from build123d import *

# Parameters (mm, degrees)
F1_DEPTH = 19.05
F2_R     = 8.5
F3_DEPTH = 3.175
F4_R     = 4.5
F5_DEPTH = 15.875
F6_R     = 8.5
F7_DEPTH = 3.175
F8_SIZE  = 0.508


with BuildPart() as f1:
    # F0 (on Front) → F1 (new body)
    with BuildSketch(Plane.XZ):
        Polygon((-30, -16), (0, -16), (30, -16), (30, 7.6738381025), (17.8103312015, 7.6746507471), (17.810886279, 16.0008126076), (0, 16.002), (-17.810886279, 16.0008126076), (-17.8103312015, 7.6746507471), (-30, 7.6738381025), align=None)
    extrude(amount=F1_DEPTH)

    # F2 (on face) → F3 (cut)
    with BuildSketch(Plane.XZ.offset(19.05)):
        Circle(F2_R)
    extrude(amount=-F3_DEPTH, mode=Mode.SUBTRACT)

    # F4 (on face) → F5 (cut, through all)
    with BuildSketch(Plane.XZ.offset(15.875)):
        Circle(F4_R)
    extrude(amount=-F5_DEPTH, mode=Mode.SUBTRACT)

    # F6 (on Front) → F7 (cut)
    with BuildSketch(Plane.XZ):
        Circle(F6_R)
    extrude(amount=F7_DEPTH, mode=Mode.SUBTRACT)

    # F8
    f8_edges = [f1.edges().sort_by_distance(p)[0] for p in [
        (-30, -9.525, 7.673838),
        (-17.810886, -9.525, 16.000813),
        (-30, -19.05, -4.163081),
        (-8.905443, -19.05, 16.001406),
        (8.905443, -19.05, 16.001406),
        (23.905166, -19.05, 7.674244),
        (30, -19.05, -4.163081),
        (0, -19.05, -16),
        (-8.905443, 0, 16.001406),
        (8.905443, 0, 16.001406),
        (17.810886, -9.525, 16.000813),
        (-30, 0, -4.163081),
        (30, 0, -4.163081),
        (0, 0, -16),
        (30, -9.525, -16),
        (-30, -9.525, -16),
        (-8.5, 0, 0),
        (-23.905166, -19.05, 7.674244),
        (-17.810609, -19.05, 11.837732),
        (17.810609, -19.05, 11.837732),
        (-8.5, -19.05, 0),
    ]]
    chamfer(f8_edges, length=F8_SIZE)


solid = f1.part
The model under review builds one solid part; all positions refer to its coordinate system, in mm. A direction names the side the tool comes from. Coordinates: 2 decimals unless noted, no trailing zeros. Loops run counter-clockwise (first coordinate to the right, second up) from the corner with the lowest first, then second, coordinate; pieces in that order, holes last. Notation, with made-up numbers: M -13.5,-21.75 L 10.5,-21.75 A24 ccw 10.5,7.25 Z; hole C -35,46 d11. An arc over 180 degrees is marked long. Put each result on its own line as item: value. Start each with the question number.
Q1. Add section B-B (z = 0). Write out the cut boundary in (x, y) (3 decimals).
Q2. Wall thickness on line 1 (Z direction, x = 0, y = -2.3); line 2 (Z direction, x = 0, y = -6); line 3 (Z direction, x = 18.5, y = -6): over which ranges is each line inside the solid? List them lowest first.
Q3. Clearance check with flat-ended pins moving along their axes: pin 1 (5 mm diameter, centred on x = 4, z = 2, fed in from -Y) (3 decimals); pin 2 (13.5 mm diameter, centred on x = -3, z = 1.5, fed in from +Y); pin 3 (8 mm diameter, centred on y = -8.5, z = 12.5, fed in from -X); pin 4 (8 mm diameter, centred on x = 0, z = 0, fed in from +Y). State where each tip first meets the part, or that it passes through.
Q4. Add section A-A (y = -6). Write out the cut boundary in (x, z), and give its area (3 significant figures).
Q5. The part is to be moulded in two halves that separate along Z. For faces 1 (the flat face through (0, -9, -16)), 2 (the flat face through (4, -15.875, -4)), 3 (the flat face through (4, -3.175, -4)), 4 (the flat face through (-30, -9, -4)), say which applies: +Z half, -Z half, draft (parallel to the pull), parting line (faces both ways), or undercut.
Q6. For faces 5 (the cylindrical face through (-0.59, -9.61, 4.46)), 6 (the cylindrical face through (4.57, -17.227, 7.167)), 7 (the cylindrical face through (4.57, -1.823, 7.167)), list the 3-axis set-ups (+Z, -Z, +X, -X, +Y, -Y) from which the entire face can be reached by the end or side of a thin tool; tool diameter is ignored.
Q7. Add section C-C (x = 26.5). Write out the cut boundary in (y, z).
Answers:
1. outline: M -30,-18.542 L -29.492,-19.05 L -9.008,-19.05 L -8.5,-18.542 L -8.5,-15.875 L -4.5,-15.875 L -4.5,-3.175 L -8.5,-3.175 L -8.5,-0.508 L -9.008,0 L -29.492,0 L -30,-0.508 Z; M 4.5,-15.875 L 8.5,-15.875 L 8.5,-18.542 L 9.008,-19.05 L 29.492,-19.05 L 30,-18.542 L 30,-0.508 L 29.492,0 L 9.008,0 L 8.5,-0.508 L 8.5,-3.175 L 4.5,-3.175 Z
2. line 1: z = -16 to -8.5, 8.5 to 16
2. line 2: z = -16 to -4.5, 4.5 to 16
2. line 3: z = -16 to 7.67
3. pin 1: stops at y = -15.875
3. pin 2: stops at y = 0
3. pin 3: stops at x = -17.81
3. pin 4: passes through
4. outline: M -30,-15.49 L -29.49,-16 L 29.49,-16 L 30,-15.49 L 30,7.67 L 17.81,7.67 L 17.81,15.49 L 17.3,16 L 0,16 L -17.3,16 L -17.81,15.49 L -17.81,7.67 L -29.49,7.67 L -30,7.17 Z; hole C 0,0 d9
4. area: 1,650 mm^2
5. face 1: -Z half
5. face 2: undercut
5. face 3: undercut
5. face 4: draft
6. face 5: +Y, -Y
6. face 6: -Y
6. face 7: +Y
7. outline: M -19.05,-15.49 L -18.54,-16 L -0.51,-16 L 0,-15.49 L 0,7.67 L -18.54,7.67 L -19.05,7.17 Z
